Source: CAD feature listing. Evaluate the final solid. Frame: model axes, mm. Face numbers are marked on the shaded views. A direction names the side the tool comes from. Give positions to 0.01 mm unless a question says otherwise; leave off trailing zeros. Order: outer loops, then holes, each group sorted by start corner. A loop starts at its lowest first (then second) coordinate and runs counter-clockwise, first axis right, second up. Notation, with made-up numbers: M -16,-1 L -11,-1 A24 ccw -11,34 Z; hole C -26.5,40.5 d5. An arc over 180 degrees is marked long. Use CSV: the item, a comma, the result in double quotes. Start each with the question number.
1. Line query: line 1 along Z through (x, y) = (0.5, 0.15); line 2 along X through (y, z) = (0.15, 0.75); line 3 along Z through (x, y) = (2.75, 0.15). Output: solid intervals per line, ascending. Write a range as [from, to].
2. Reachability of the marked faces 1 and 2 from +Z, -Z, +X, -X, +Y, -Y: full face, straight path, thin tool, end or side. Return the list, or none.
3. Section query C-C, the plane y = 0.15. Return the cut outline in (x, z), plus the area to 3 significant figures.
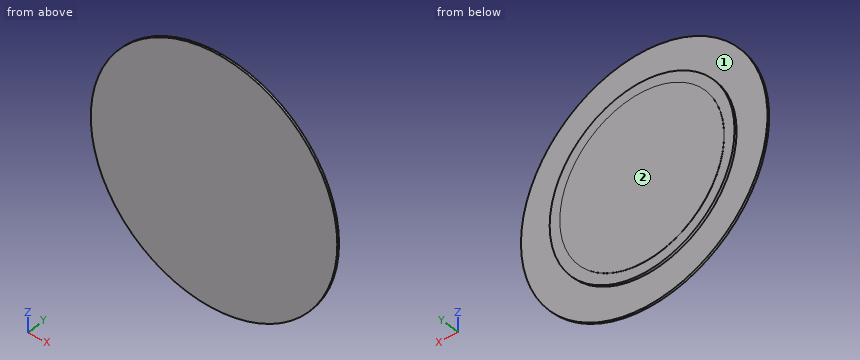
from build123d import *

# Parameters (mm, degrees)
SKETCH_1_R      = 6
EXTRUDE_1_DEPTH = 0.1
SKETCH_2_R      = 4.5
EXTRUDE_2_DEPTH = 0.12
SKETCH_3_R      = 4
EXTRUDE_3_DEPTH = 0.01


with BuildPart() as part:
    # 草图1 → 凸台-拉伸1 (new body)
    with BuildSketch(Plane(origin=(0, 0, 0), x_dir=(1, 0, 0), z_dir=(0, 1, 0))):
        Circle(SKETCH_1_R)
    extrude(amount=EXTRUDE_1_DEPTH)

    # 草图2 → 凸台-拉伸2 (add)
    with BuildSketch(Plane(origin=(0, 0.1, 0), x_dir=(1, 0, 0), z_dir=(0, 1, 0))):
        Circle(SKETCH_2_R)
    extrude(amount=EXTRUDE_2_DEPTH)

    # 草图3 → 凸台-拉伸3 (add)
    with BuildSketch(Plane(origin=(0, 0.22, 0), x_dir=(1, 0, 0), z_dir=(0, 1, 0))):
        Circle(SKETCH_3_R)
    extrude(amount=EXTRUDE_3_DEPTH)


solid = part.part
Result set:
1,line 1,"[-4.47, 4.47]"
1,line 2,"[-4.44, 4.44]"
1,line 3,"[-3.56, 3.56]"
2,face 1,"+Y"
2,face 2,"+Z, -Z, +X, -X, +Y"
3,outline,"C 0,0 d9"
3,area,"63.6 mm2"
